Input: dimensioned drawing with shaded views. Units: mm. Origin: part minimum x, y, z. Give positions to 0.01 mm unless a question says otherwise; leave off trailing zeros. Write each loop counter-clockwise with the first axis right and the second up, starting at its lowest first coordinate (ties: lowest second). Pieces come first, ordered by that corner, then holes. Notation, with made-up numbers: (39.5, 53) - (63.5, 53) arc R18 cw to (63.5, 77) - close; hole circle Ø10 at (66.5, -6). An arc over 180 degrees is marked (long way). Answer as a JSON object with one key per item and string values. Group by question number.
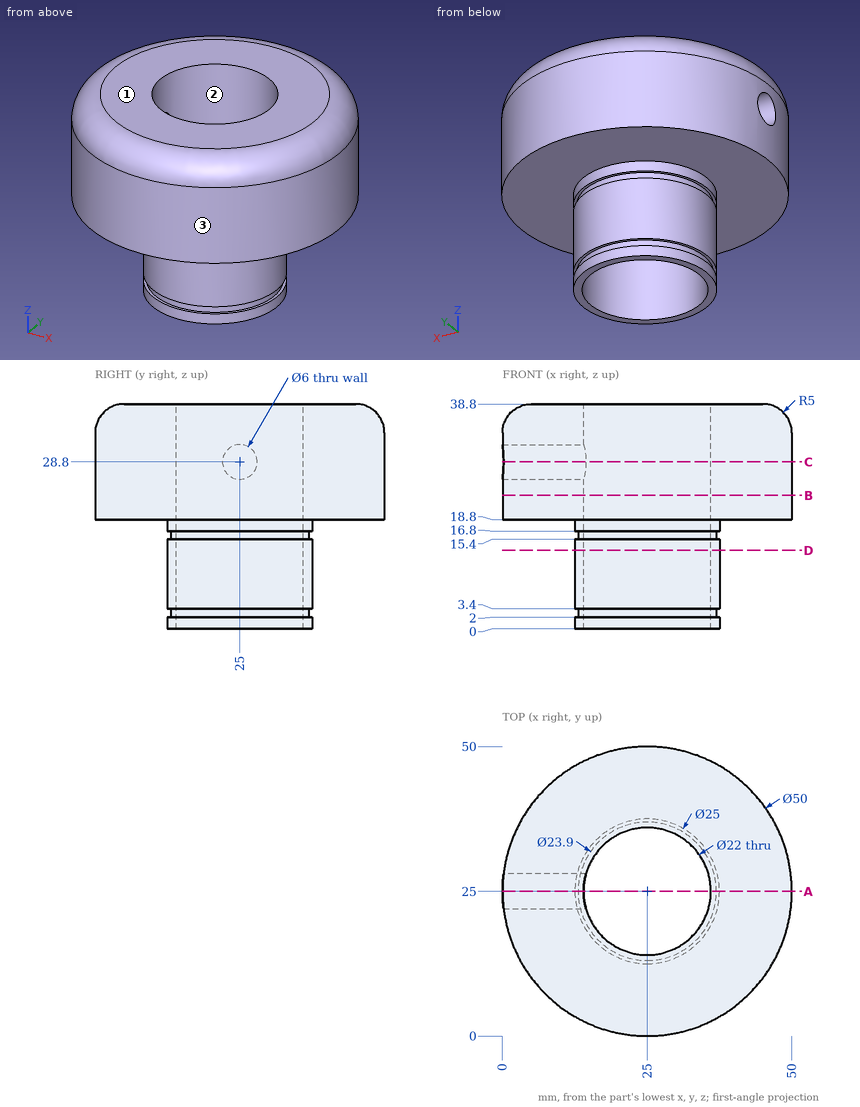
1) Cut plane D-D on z = 13.5. Return the cut outline in (x, y).
2) Cut plane B-B on z = 23. Return the cut outline in (x, y), and give its area (3 significant figures).
3) Mould query, pull axis X, two halves, no side actions, for the marked faces 1, 2 and 3. Classes: +X half, -X half, draft (parallel to the pull), parting line (faces both ways), or undercut.
4) Pin query (flat end, axial travel): P1, Ø6, axis at x = 17.5, z = 5.5, coming from the +Y side; P2, Ø1, axis at x = 39, y = 13.5, coming from the -Z side; P3, Ø2, axis at x = 36.5, z = 7, coming from the -Y side; P4, Ø7.5, axis at x = 22.5, y = 20.5, coming from the +Z side. Return the tip coordinate at first contact, or that it passes through.
5) Line query: line 1 along Z through (x, y) = (5, 25); line 2 along X through (y, z) = (25, 14); line 3 along Z through (x, y) = (13.5, 36). Output: solid intervals per line, ascending. Write a range as from..to.
6) Cut plane C-C on z = 28.8. Return the cut outline in (x, y), and give its area (3 significant figures).
7) Cut plane A-A on y = 25. Count the separate pieces of the cut face and the enclosed holes in it, and give its area (3 significant figures).
Filled in:
{
 "1": {"outline": "circle Ø25 at (25, 25); hole circle Ø22 at (25, 25)"},
 "2": {"outline": "circle Ø50 at (25, 25); hole circle Ø22 at (25, 25)", "area": "1,580 mm²"},
 "3": {"face 1": "draft", "face 2": "undercut", "face 3": "parting line"},
 "4": {"P1": "stops at y = 36.66", "P2": "stops at z = 18.8", "P3": "stops at y = 18.22", "P4": "passes through"},
 "5": {"line 1": "z = 18.8..25.8, 31.8..38.8", "line 2": "x = 12.5..14, 36..37.5", "line 3": "z = 18.8..38.8"},
 "6": {"outline": "(0.18, 22) arc R25 ccw (long way) to (0.18, 28) - (14.42, 28) arc R11 cw (long way) to (14.42, 22) - close", "area": "1,500 mm²"},
 "7": {"separate pieces": "3", "enclosed holes": "0", "area": "519 mm²"}
}
